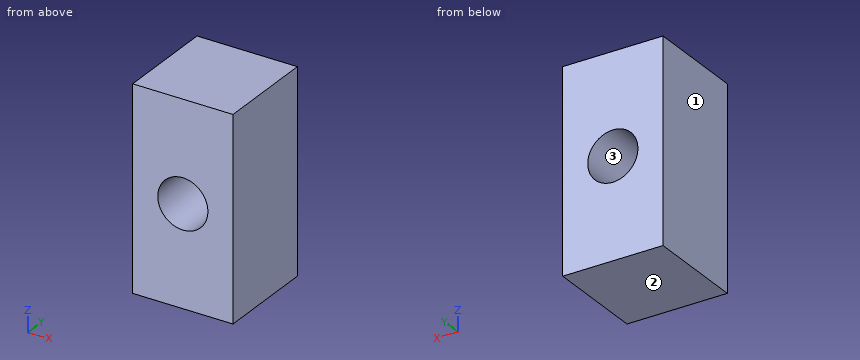
```python
from build123d import *

# Parameters (mm, degrees)
SKETCH1_W           = 25.4
SKETCH1_H           = 50.8
BOSS_EXTRUDE1_DEPTH = 25.4
CUT_EXTRUDE1_REACH  = 27.4
SKETCH2_R           = 6.35


with BuildPart() as part:
    # Sketch1 → Boss-Extrude1 (new body)
    with BuildSketch(Plane(origin=(0, 0, 0), x_dir=(1, 0, 0), z_dir=(0, 1, 0))):
        Rectangle(SKETCH1_W, SKETCH1_H)
    extrude(amount=BOSS_EXTRUDE1_DEPTH)

    # Sketch2 → Cut-Extrude1 (cut, up to next)
    with BuildSketch(Plane(origin=(0, 25.4, 0), x_dir=(1, 0, 0), z_dir=(0, 1, 0)), mode=Mode.PRIVATE) as cut_extrude1_sk1:
        Circle(SKETCH2_R)
    cut_extrude1_tool1 = extrude(cut_extrude1_sk1.sketch, amount=-CUT_EXTRUDE1_REACH, mode=Mode.PRIVATE) & part.part
    add(cut_extrude1_tool1.solids().sort_by_distance((0, 25.4, 0))[0], mode=Mode.SUBTRACT)


solid = part.part
```
CAD build for the part. Positions are in the model's coordinates, mm. Face numbers are marked on the shaded views. Round coordinates to 2 decimals unless told otherwise and drop trailing zeros. Order: outer loops, then holes, each group sorted by start corner. A loop starts at its lowest first (then second) coordinate and runs counter-clockwise, first axis right, second up. Notation, with made-up numbers: (6.25, 26) - (34.25, 26) arc R24 ccw to (34.25, 42) - close; hole circle Ø1 at (67.5, 7.5). An arc over 180 degrees is marked (long way). Answer as CSV lines item,"result". Start each with the question number.
1. Pin check, flat tip, straight feed: pin 1 (11.5 mm diameter, centred on x = 0, z = 0, fed in from -Y). Stop position of the tip, or through.
2. Saw through at A-A, the plane z = 0. Write the cut outline in (x, y), and give its area (3 significant figures).
3. Saw through at B-B, the plane x = 0. Write the cut outline in (y, z).
4. Pull direction X, two halves, no side cores. Call the marked faces 1, 2 and 3: +X half, -X half, draft (parallel to the pull), parting line (faces both ways), or undercut.
5. Saw through at C-C, the plane y = 2.75. Write the cut outline in (x, z).
6. Drill centre lines: L1, parallel to X at y = 8.25, z = 0; L2, parallel to Z at x = 0, y = 9.25; L3, parallel to X at y = 16, z = -3. Where is each one in solid material? Low to high. Write a range as [from, to].
Model answer:
1,pin 1,"passes through"
2,outline,"(-12.7, 0) - (-6.35, 0) - (-6.35, 25.4) - (-12.7, 25.4) - close; (6.35, 0) - (12.7, 0) - (12.7, 25.4) - (6.35, 25.4) - close"
2,area,"323 mm²"
3,outline,"(0, -25.4) - (25.4, -25.4) - (25.4, -6.35) - (0, -6.35) - close; (0, 6.35) - (25.4, 6.35) - (25.4, 25.4) - (0, 25.4) - close"
4,face 1,"-X half"
4,face 2,"draft"
4,face 3,"undercut"
5,outline,"(-12.7, -25.4) - (12.7, -25.4) - (12.7, 25.4) - (-12.7, 25.4) - close; hole circle Ø12.7 at (0, 0)"
6,L1,"x = [-12.7, -6.35], [6.35, 12.7]"
6,L2,"z = [-25.4, -6.35], [6.35, 25.4]"
6,L3,"x = [-12.7, -5.6], [5.6, 12.7]"
